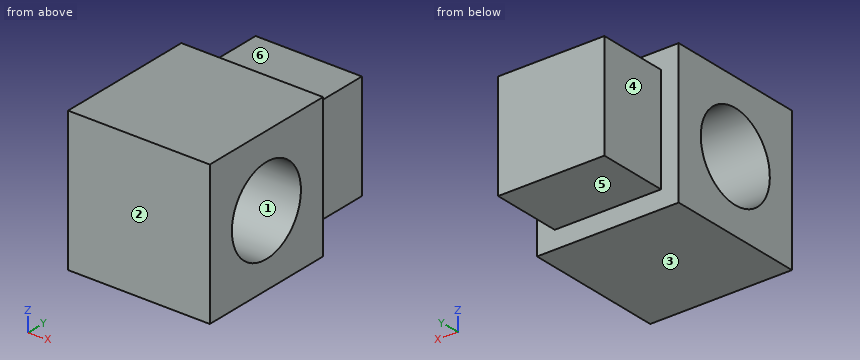
```python
from build123d import *

# Parameters (mm, degrees)
SKETCH1_W           = 20
SKETCH1_H           = 20
SKETCH1_R           = 6.1
BOSS_EXTRUDE1_DEPTH = 10
SKETCH3_W           = 15
SKETCH3_H           = 15
BOSS_EXTRUDE2_DEPTH = 10


with BuildPart() as part:
    # Sketch1 → Boss-Extrude1 (new body, symmetric)
    with BuildSketch(Plane(origin=(0, 0, 0), x_dir=(0, 0, -1), z_dir=(1, 0, 0))):
        Rectangle(SKETCH1_W, SKETCH1_H)
        Circle(SKETCH1_R, mode=Mode.SUBTRACT)
    extrude(amount=BOSS_EXTRUDE1_DEPTH, both=True)

    # Sketch3 → Boss-Extrude2 (add)
    with BuildSketch(Plane(origin=(0, 10, 0), x_dir=(1, 0, 0), z_dir=(0, 1, 0))):
        Rectangle(SKETCH3_W, SKETCH3_H)
    extrude(amount=BOSS_EXTRUDE2_DEPTH)


solid = part.part
```
Geometry check sheet. Reference: the model listing, model coordinates, mm. Face numbers are marked on the shaded views. A direction names the side the tool comes from. Coordinates: 2 decimals unless noted, no trailing zeros. Order: outer loops, then holes, each group sorted by start corner. A loop starts at its lowest first (then second) coordinate and runs counter-clockwise, first axis right, second up.
Q1. Depth check by flat-ended pin: pin 1 Ø5 at (y, z) = (16.5, -2.5) entering from +X; pin 2 Ø5 at (x, y) = (2.5, 16) entering from +Z. Enter the tip coordinate at first touch or a pass-through.
Reply:
pin 1: stops at x = 7.5
pin 2: stops at z = 7.5
Q2. Thickness scan on probe 1 along Y at (x, z) = (-2, 0); probe 2 along X at (y, z) = (13.5, 1); probe 3 along Z at (x, y) = (-5, 0.25). Record the ranges inside material, lowest first.
Reply:
probe 1: y = -10 to -6.1, 6.1 to 20
probe 2: x = -7.5 to 7.5
probe 3: z = -10 to -6.09, 6.09 to 10
Q3. Sectioned sample at B-B on y = 0. Record the cut outline in (x, z).
Reply:
outline: (-10, -10) - (10, -10) - (10, -6.1) - (-10, -6.1) - close; (-10, 6.1) - (10, 6.1) - (10, 10) - (-10, 10) - close
Q4. Tool access check on the marked faces 4, 5 and 6. Record the directions out of +Z, -Z, +X, -X, +Y, -Y that give a thin tool (end or side, any length) a straight path to the whole face; none if there is none.
Reply:
face 4: +Z, -Z, -X, +Y
face 5: -Z, +X, -X, +Y
face 6: +Z, +X, -X, +Y
Q5. Sectioned sample at A-A on x = -6.75. Record the cut outline in (y, z), and give its area (3 significant figures).
Reply:
outline: (-10, -10) - (10, -10) - (10, -7.5) - (20, -7.5) - (20, 7.5) - (10, 7.5) - (10, 10) - (-10, 10) - close; hole circle Ø12.2 at (0, 0)
area: 433 mm2
Q6. Sectioned sample at C-C on z = 0. Record the cut outline in (x, y), and give its area (3 significant figures).
Reply:
outline: (-10, -10) - (10, -10) - (10, -6.1) - (-10, -6.1) - close; (-10, 6.1) - (10, 6.1) - (10, 10) - (7.5, 10) - (7.5, 20) - (-7.5, 20) - (-7.5, 10) - (-10, 10) - close
area: 306 mm2
Q7. Draft check along Z on the marked faces 1, 2 and 3. Enter one of: released by +Z, released by -Z, zero draft, split by the parting line, or undercut.
Reply:
face 1: undercut
face 2: zero draft
face 3: released by -Z
Q8. Sectioned sample at D-D on z = -3.25. Record the cut outline in (x, y).
Reply:
outline: (-10, -10) - (10, -10) - (10, -5.16) - (-10, -5.16) - close; (-10, 5.16) - (10, 5.16) - (10, 10) - (7.5, 10) - (7.5, 20) - (-7.5, 20) - (-7.5, 10) - (-10, 10) - close
